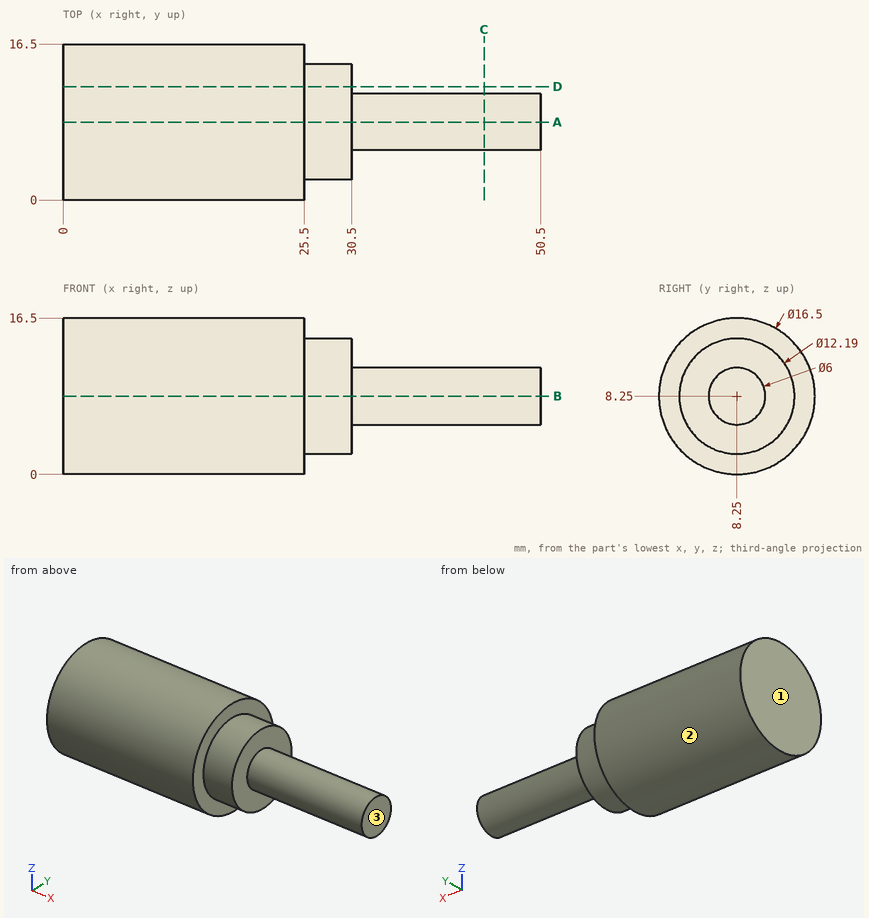
Could you check a few things on this drawing? It's one solid part, dimensions in mm from its lowest x, y, z. Coordinates: 2 decimals unless noted, no trailing zeros. Loops run counter-clockwise (first coordinate to the right, second up) from the corner with the lowest first, then second, coordinate; pieces in that order, holes last.
1. We'd pull the mould along X, two halves only. Please class the marked faces 1, 2 and 3: released by +X, released by -X, zero draft, split by the parting line, or undercut.
2. Imagine slicing it at C-C (x = 44.5). Please give me the cut outline in (y, z), and give its area (3 significant figures).
3. Imagine slicing it at D-D (y = 12). Please give me the cut outline in (x, z).
4. Imagine slicing it at A-A (y = 8.25). Please give me the cut outline in (x, z) (3 decimals).
5. I need wall thicknesses on L1, parallel to X at y = 14, z = 5; L2, parallel to Y at x = 5, z = 8; L3, parallel to X at y = 8.75, z = 2.5. Which ranges of each line are inside material? Lowest first, please.
6. For P1, Ø4, axis at x = 26, y = 9, coming from the -Z side; P2, Ø4, axis at x = 40.5, z = 7.5, coming from the -Y side; P3, Ø1, axis at x = 40, y = 11, coming from the +Z side; P4, Ø5, axis at x = 28.5, y = 9.5, coming from the +Z side (3 decimals), each with a flat end and sliding along its axis, tell me the tip position at first contact or that it passes through.
Computed values:
1. face 1: released by -X
1. face 2: zero draft
1. face 3: released by +X
2. outline: circle Ø6 at (8.25, 8.25)
2. area: 28.3 mm2
3. outline: (0, 0.9) - (25.5, 0.9) - (25.5, 3.45) - (30.5, 3.45) - (30.5, 13.05) - (25.5, 13.05) - (25.5, 15.6) - (0, 15.6) - close
4. outline: (0, 0) - (25.5, 0) - (25.5, 2.155) - (30.5, 2.155) - (30.5, 5.25) - (50.5, 5.25) - (50.5, 11.25) - (30.5, 11.25) - (30.5, 14.345) - (25.5, 14.345) - (25.5, 16.5) - (0, 16.5) - close
5. L1: x = 0 to 25.5
5. L2: y = 0 to 16.5
5. L3: x = 0 to 30.5
6. P1: stops at z = 0
6. P2: stops at y = 5.25
6. P3: stops at z = 10.23
6. P4: stops at z = 14.345
